Part model, mm, in its own coordinate system. Face numbers are marked on the shaded views. A direction names the side the tool comes from. Round coordinates to 2 decimals unless told otherwise and drop trailing zeros. Loops run counter-clockwise (first coordinate to the right, second up) from the corner with the lowest first, then second, coordinate; pieces in that order, holes last. Notation, with made-up numbers: (16.5, 87) - (26.5, 87) arc R21 ccw to (26.5, 126) - close; hole circle Ø3 at (11.5, -12.5). An arc over 180 degrees is marked (long way). Put each result on its own line as item: value.
from build123d import *

# Parameters (mm, degrees)
SKETCH_1_R      = 6
EXTRUDE_1_DEPTH = 6
EXTRUDE_START   = -20
EXTRUDE_2_DEPTH = 20
FILLET_1_R      = 4


with BuildPart() as part:
    # Эскиз1 → Бобышка-Вытянуть1 (new body)
    with BuildSketch(Plane.XY):
        with BuildLine():
            Line((-40, 0), (-6, 0))
            ThreePointArc((-6, 0), (-1.757359313, -1.757359313), (0, -6))
            Line((0, -6), (0, -20))
            Line((0, -20), (10.931919214, -20))
            Line((10.931919214, -20), (31.276311449, 35.89575828))
            ThreePointArc((31.276311449, 35.89575828), (27.305137148, 49.520240083), (13.117082764, 49.829824531))
            Line((13.117082764, 49.829824531), (-40, 12.636842773))
            Line((-40, 12.636842773), (-40, 0))
        make_face()
        with Locations((20, 40)):
            Circle(SKETCH_1_R, mode=Mode.SUBTRACT)
    extrude(amount=EXTRUDE_1_DEPTH)

    # Эскиз2 → Бобышка-Вытянуть2 (add)
    with BuildSketch(Plane.XY.offset(EXTRUDE_START)):
        with BuildLine():
            Line((-40, 0), (-6, 0))
            ThreePointArc((-6, 0), (-1.757359313, -1.757359313), (0, -6))
            Line((0, -6), (0, -20))
            Line((0, -20), (6, -20))
            Line((6, -20), (6, -6))
            ThreePointArc((6, -6), (2.485281374, 2.485281374), (-6, 6))
            Line((-6, 6), (-40, 6))
            Line((-40, 6), (-40, 0))
        make_face()
    extrude(amount=EXTRUDE_2_DEPTH)

    # Скругление1
    fillet_1_edges = [part.edges().sort_by_distance(p)[0] for p in [
        (6, -13, 0),
        (2.485281374, 2.485281374, 0),
        (-23, 6, 0),
    ]]
    fillet(fillet_1_edges, radius=FILLET_1_R)


solid = part.part
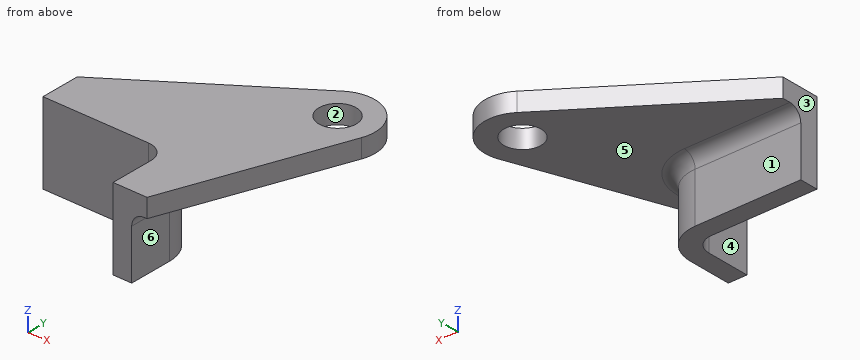
1. Band-saw the part on B-B (z = -6.5). List the corners of the cut face in (x, y), plus the area to 3 significant figures.
A:
outline: (-40, 0) - (-6, 0) arc R6 cw to (0, -6) - (0, -20) - (6, -20) - (6, -6) arc R12 ccw to (-6, 6) - (-40, 6) - close
area: 373 mm²
2. Probe line 1 along Z through (x, y) = (28, 27.5). List the from-to ranges inside material, lowest first. Write a range as [from, to].
A:
line 1: z = [0, 6]
3. Two-plate mould, pull along Y, no slides. Class the marked faces 1, 2 and 3: pulls with the +Y half, pulls with the -Y half, needs draft (parallel to the pull), parting line crosses it, or undercut.
A:
face 1: pulls with the +Y half
face 2: undercut
face 3: needs draft
4. Band-saw the part on D-D (x = -32.5). List the corners of the cut face in (y, z).
A:
outline: (0, -20) - (6, -20) - (6, -4) arc R4 cw to (10, 0) - (17.89, 0) - (17.89, 6) - (0, 6) - close
5. Band-saw the part on C-C (y = 40). List the corners of the cut face in (x, z), plus the area to 3 significant figures.
A:
outline: (-0.92, 0) - (14, 0) - (14, 6) - (-0.92, 6) - close; (26, 0) - (32, 0) - (32, 6) - (26, 6) - close
area: 126 mm²
6. Pin check, flat tips, straight feed: P1, Ø1, axis at x = 10, y = 36.5, coming from the -Z side; P2, Ø7, axis at x = 20, y = 40, coming from the -Z side (1 decimal); P3, Ø13, axis at x = -30.5, z = -3.5, coming from the -Y side; P4, Ø1, axis at x = -31, z = -9, coming from the +Y side. Stop position of each tip, or through.
A:
P1: stops at z = 0
P2: passes through
P3: stops at y = 0
P4: stops at y = 6
7. Tool access for the marked faces 4, 5 and 6: list every direction of +Z, -Z, +X, -X, +Y, -Y with a clear straight run to the whole face (end or side of a thin tool).
A:
face 4: +Z, -Z, -X, -Y
face 5: -Z, +X, +Y
face 6: -Z, +X, +Y, -Y
8. Band-saw the part on A-A (x = 20). List the corners of the cut face in (y, z).
A:
outline: (4.91, 0) - (34, 0) - (34, 6) - (4.91, 6) - close; (46, 0) - (52, 0) - (52, 6) - (46, 6) - close
